Build history of the part. All positions in model axes, mm. A direction names the side the tool comes from. Give positions to 0.01 mm unless a question says otherwise; leave off trailing zeros. Write each loop counter-clockwise with the first axis right and the second up, starting at its lowest first coordinate (ties: lowest second). Pieces come first, ordered by that corner, then holes. Notation, with made-up numbers: (41, 77) -> (84, 77) arc R21 ccw to (84, 95) -> close; hole circle Ø9 at (-28, 33). An arc over 180 degrees is marked (long way). One line per question, with ' | ' between items. Start each with the question number.
(1) Drill centre lines: probe 1 along X at (y, z) = (5.25, -3); probe 2 along X at (y, z) = (1, -38.5); probe 3 along Z at (x, y) = (19.5, 7). Where is each one in solid material? Low to high. Write a range as from..to.
(2) Pin check, flat tips, straight feed: P1, Ø1.8, axis at x = 45, z = -45, coming from the +Y side; P2, Ø3, axis at x = 47, z = -26.5, coming from the -Y side; P3, Ø1.8, axis at x = 46.5, y = 2, coming from the -Z side. Stop position of each tip, or through.
(3) Band-saw the part on B-B, the plane y = 2. Give the cut face in (x, z), and give its area (4 significant figures).
(4) Band-saw the part on D-D, the plane y = 8.75. Give the cut face in (x, z), and give its area (4 significant figures).
(5) Band-saw the part on C-C, the plane x = 32. Give the cut face in (y, z).
(6) Pull direction X, two halves, no side cores. Call faces 4 (the cylindrical face through (3.07, 5.92, -46.5)), 5 (the flat face through (3, 0, -22)), 6 (the cylindrical face through (0.9, 5.92, -47.14)): released by +X, released by -X, zero draft, split by the parting line, or undercut.
(7) Tool access for faces 1 (the cylindrical face through (0.86, 5.92, -0.9)), 2 (the flat face through (5.3, 5.9, -5.2)), 3 (the flat face through (46, 2, -34)): list every direction of +Z, -Z, +X, -X, +Y, -Y with a clear straight run to the whole face (end or side of a thin tool).
(8) Band-saw the part on A-A, the plane z = -42.5. Give the cut face in (x, y).
from build123d import *

# Parameters (mm, degrees)
SKETCH3_R           = 1.5
BOSS_EXTRUDE1_DEPTH = 12
SKETCH4_W           = 20
SKETCH4_H           = 3.5
CUT_EXTRUDE1_DEPTH  = 4


with BuildPart() as part:
    # Sketch3 → Boss-Extrude1 (new body)
    with BuildSketch(Plane(origin=(0, 0, 0), x_dir=(1, 0, 0), z_dir=(0, 1, 0))):
        with BuildLine():
            Line((3, 0), (45, 0))
            ThreePointArc((45, 0), (47.121320344, 0.878679656), (48, 3))
            Line((48, 3), (48, 45))
            ThreePointArc((48, 45), (47.121320344, 47.121320344), (45, 48))
            Line((45, 48), (3, 48))
            ThreePointArc((3, 48), (0.878679656, 47.121320344), (0, 45))
            Line((0, 45), (0, 3))
            ThreePointArc((0, 3), (0.878679656, 0.878679656), (3, 0))
        make_face()
        with Locations(Location((3, 45, 0), (0, 0, 270))):
            Circle(SKETCH3_R, mode=Mode.SUBTRACT)
        with Locations(Location((3, 3, 0), (0, 0, 90))):
            Circle(SKETCH3_R, mode=Mode.SUBTRACT)
        with Locations(Location((45, 3, 0), (0, 0, 270))):
            Circle(SKETCH3_R, mode=Mode.SUBTRACT)
        with Locations(Location((45, 45, 0), (0, 0, 90))):
            Circle(SKETCH3_R, mode=Mode.SUBTRACT)
        Polygon((4, 41.5), (6.5, 44), (41.5, 44), (44, 41.5), (44, 6.5), (41.5, 4), (6.5, 4), (4, 6.5), align=None, mode=Mode.SUBTRACT)
    extrude(amount=BOSS_EXTRUDE1_DEPTH)

    # Sketch4 → Cut-Extrude1 (cut)
    with BuildSketch(Plane(origin=(48, 0, 0), x_dir=(0, 0, -1), z_dir=(1, 0, 0))):
        with Locations((24, 1.75)):
            Rectangle(SKETCH4_W, SKETCH4_H)
    extrude(amount=-CUT_EXTRUDE1_DEPTH, mode=Mode.SUBTRACT)


solid = part.part
Results:
1) probe 1: x = 0..1.5, 4.5..43.5, 46.5..48 | probe 2: x = 0..4, 44..48 | probe 3: z = -48..-44, -4..0
2) P1: passes through | P2: stops at y = 3.5 | P3: stops at z = -47.94
3) outline: (0, -45) arc R3 ccw to (3, -48) -> (45, -48) arc R3 ccw to (48, -45) -> (48, -34) -> (44, -34) -> (44, -41.5) -> (41.5, -44) -> (6.5, -44) -> (4, -41.5) -> (4, -6.5) -> (6.5, -4) -> (41.5, -4) -> (44, -6.5) -> (44, -14) -> (48, -14) -> (48, -3) arc R3 ccw to (45, 0) -> (3, 0) arc R3 ccw to (0, -3) -> close; hole circle Ø3 at (3, -45); hole circle Ø3 at (3, -3); hole circle Ø3 at (45, -45); hole circle Ø3 at (45, -3) | area: 600.5 mm²
4) outline: (0, -45) arc R3 ccw to (3, -48) -> (45, -48) arc R3 ccw to (48, -45) -> (48, -3) arc R3 ccw to (45, 0) -> (3, 0) arc R3 ccw to (0, -3) -> close; hole circle Ø3 at (3, -45); hole circle Ø3 at (3, -3); hole (4, -41.5) -> (6.5, -44) -> (41.5, -44) -> (44, -41.5) -> (44, -6.5) -> (41.5, -4) -> (6.5, -4) -> (4, -6.5) -> close; hole circle Ø3 at (45, -45); hole circle Ø3 at (45, -3) | area: 680.5 mm²
5) outline: (0, -48) -> (12, -48) -> (12, -44) -> (0, -44) -> close; (0, -4) -> (12, -4) -> (12, 0) -> (0, 0) -> close
6) face 4: undercut | face 5: zero draft | face 6: released by -X
7) face 1: +Z, -X, +Y, -Y | face 2: +Y, -Y | face 3: +X, -Y
8) outline: (0, 0) -> (5, 0) -> (5, 12) -> (0, 12) -> close; (43, 0) -> (48, 0) -> (48, 12) -> (43, 12) -> close
